Model file for the job. Use its own axes, mm. A direction names the side the tool comes from. Coordinates: 2 decimals unless noted, no trailing zeros. Order: outer loops, then holes, each group sorted by start corner. A loop starts at its lowest first (then second) coordinate and runs counter-clockwise, first axis right, second up.
from build123d import *

# Parameters (mm, degrees)
F0_W      = 38.1
F0_H      = 76.2
F1_DEPTH  = 177.8
F2_W      = 76.2
F2_H      = 25.4
F3_DEPTH  = 25.4
F5_DEPTH  = 25.4
F7_DEPTH  = 25.4
F8_W      = 38.1
F8_H      = 76.2
F9_DEPTH  = 25.4
F10_W     = 25.4
F10_H     = 25.4
F11_DEPTH = 228.6
F12_W     = 76.2
F12_H     = 50.8
F13_DEPTH = 38.1
F15_DEPTH = 228.6


with BuildPart() as f1:
    # F0 (on Top) → F1 (new body)
    with BuildSketch(Plane.XY):
        Rectangle(F0_W, F0_H)
    extrude(amount=F1_DEPTH)

    # F2 (on face) → F3 (join)
    with BuildSketch(Plane(origin=(-19.05, 0, 0), x_dir=(0, -1, 0), z_dir=(-1, 0, 0))):
        with Locations((0, 127)):
            Rectangle(F2_W, F2_H)
    extrude(amount=F3_DEPTH)

    # F4 (on face) → F5 (join)
    with BuildSketch(Plane.XZ.offset(38.1)):
        Polygon((-44.45, 139.7), (-44.45, 114.3), (-19.05, 114.3), (19.05, 114.3), (19.05, 139.7), (-19.05, 139.7), align=None)
    extrude(amount=F5_DEPTH)

    # F6 (on face) → F7 (join)
    with BuildSketch(Plane(origin=(0, 38.1, 0), x_dir=(-1, 0, 0), z_dir=(0, 1, 0))):
        Polygon((44.45, 114.3), (44.45, 139.7), (19.05, 139.7), (-19.05, 139.7), (-19.05, 114.3), (19.05, 114.3), align=None)
    extrude(amount=F7_DEPTH)

    # F8 (on face) → F9 (join)
    with BuildSketch(Plane.XY.offset(177.8)):
        Rectangle(F8_W, F8_H)
    extrude(amount=F9_DEPTH)

    # F10 (on face) → F11 (cut)
    with BuildSketch(Plane.XY.offset(203.2)):
        Rectangle(F10_W, F10_H)
    extrude(amount=-F11_DEPTH, mode=Mode.SUBTRACT)

    # F12 (on face) → F13 (join)
    with BuildSketch(Plane.YZ.offset(19.05)):
        with Locations((0, 25.4)):
            Rectangle(F12_W, F12_H)
    extrude(amount=F13_DEPTH)

    # F14 (on face) → F15 (cut)
    with BuildSketch(Plane.XZ.offset(38.1)):
        with BuildLine():
            Line((38.1, 50.8), (19.05, 50.8))
            ThreePointArc((19.05, 50.8), (28.575, 49.590166), (38.1, 50.8))
        make_face()
    extrude(amount=-F15_DEPTH, mode=Mode.SUBTRACT)


solid = f1.part
Q1. Cut at A-A, the plane z = 40. List the corners of the cut face in (x, y), plus the area to 3 significant figures.
Established:
outline: (-19.05, -38.1) - (57.15, -38.1) - (57.15, 38.1) - (-19.05, 38.1) - close; hole (-12.7, -12.7) - (12.7, -12.7) - (12.7, 12.7) - (-12.7, 12.7) - close
area: 5,160 mm2
Q2. Probe line 1 (Y direction, x = -10.5, z = 140); line 2 (X direction, y = -2, z = 94.5); line 3 (X direction, y = -19, z = 17). List the from-to ranges inside material, lowest first.
Established:
line 1: y = -38.1 to -12.7, 12.7 to 38.1
line 2: x = -19.05 to -12.7, 12.7 to 19.05
line 3: x = -19.05 to 57.15
Q3. Cut at D-D, the plane z = 106.5. List the corners of the cut face in (x, y), plus the area to 3 significant figures.
Established:
outline: (-19.05, -38.1) - (19.05, -38.1) - (19.05, 38.1) - (-19.05, 38.1) - close; hole (-12.7, -12.7) - (12.7, -12.7) - (12.7, 12.7) - (-12.7, 12.7) - close
area: 2,260 mm2
Q4. Drop flat-ended pins along their axis: P1, Ø12, axis at y = -17, z = 104, coming from the +X side; P2, Ø5.5, axis at x = 51, y = -12.5, coming from the +Z side; P3, Ø2, axis at x = 12, z = 45.5, coming from the +Y side; P4, Ø10, axis at x = 27.5, z = 59, coming from the -Y side. Give the stop position or say it passes through.
Established:
P1: stops at x = 19.05
P2: stops at z = 50.8
P3: stops at y = 38.1
P4: passes through
Q5. Cut at B-B, the plane y = -7. List the corners of the cut face in (x, z) (3 decimals), plus the area to 3 significant figures.
Established:
outline: (-44.45, 114.3) - (-19.05, 114.3) - (-19.05, 0) - (-12.7, 0) - (-12.7, 203.2) - (-19.05, 203.2) - (-19.05, 139.7) - (-44.45, 139.7) - close; (12.7, 0) - (57.15, 0) - (57.15, 50.8) - (38.1, 50.8) arc R38.1 cw to (19.05, 50.8) - (19.05, 203.2) - (12.7, 203.2) - close
area: 5,150 mm2
Q6. Cut at C-C, the plane x = -5.5. List the corners of the cut face in (y, z).
Established:
outline: (-63.5, 114.3) - (-38.1, 114.3) - (-38.1, 0) - (-12.7, 0) - (-12.7, 203.2) - (-38.1, 203.2) - (-38.1, 139.7) - (-63.5, 139.7) - close; (12.7, 0) - (38.1, 0) - (38.1, 114.3) - (63.5, 114.3) - (63.5, 139.7) - (38.1, 139.7) - (38.1, 203.2) - (12.7, 203.2) - close
Q7. Mould opens along Y. For faces 4 (the face through (12.7, 0, 103)), 5 (the face through (10, -38.1, 44)), 6 (the face through (-13, 1, 203.2)) say: pulls with the +Y half, pulls with the -Y half, needs draft (parallel to the pull), parting line crosses it, or undercut.
Established:
face 4: undercut
face 5: pulls with the -Y half
face 6: needs draft
Q8. Which spindle directions (+Z, -Z, +X, -X, +Y, -Y) get a long thin tool onto all of the face, cutting with end or side? Do faces 1 (the face through (19.05, -1, 126)), 2 (the face through (-12.7, 0, 103)), 3 (the face through (-19.05, -1, 171)). Say none if no direction does.
Established:
face 1: +Z, +X, +Y, -Y
face 2: +Z, -Z
face 3: +Z, -X, +Y, -Y
